Answer from the drawing. Dimensions are ordinates in mm from the lowest x, y and z of the part. A direction names the side the tool comes from. Round coordinates to 2 decimals unless told otherwise and drop trailing zeros. Loops run counter-clockwise (first coordinate to the right, second up) from the corner with the lowest first, then second, coordinate; pieces in that order, holes last. Notation, with made-up numbers: (-40, -29.75) - (-18, -29.75) arc R29 cw to (-18, -6.75) - close; hole circle Ø9 at (-27, 18.25). An arc over 180 degrees is marked (long way). Write item = value, one per line. Start each with the question number.
1) For a pull along X with two mould halves and no side action, classify the marked faces 1, 2, 3 and 4 as released by +X, released by -X, zero draft, split by the parting line, or undercut.
2) Section D-D, the plane y = 23.5 is taken. Determine the outline of the cut face in (x, z).
3) A tool of negligible diameter and unlimited length cuts with its end or side. For the marked faces 5 and 6, from which of +Z, -Z, +X, -X, +Y, -Y can it reach the whole face along a straight path? Write none if from no direction.
4) Given pin 1 Ø1.5 at (x, z) = (55, 13.5) entering from -Y; pin 2 Ø10 at (y, z) = (11.5, 63) entering from +X; pin 3 Ø2 at (y, z) = (15.5, 43.5) entering from +X (1 decimal), each flat-ended and moving along its own axis, determine where each tip first touches the part or whether it passes through.
5) Straight lines are drawn through the part: line 1 along Z through (x, y) = (50.8, 34.5); line 2 along Z through (x, y) = (50.8, 15.5); line 3 along Y through (x, z) = (118, 14.5). For each, find the intervals that lie inside material, in ascending order.
6) Section B-B, the plane x = 27 is taken. Determine the outline of the cut face in (y, z).
7) Section C-C, the plane y = 41.5 is taken. Determine the outline of the cut face in (x, z).
8) Section A-A, the plane z = 50.8 is taken. Determine the outline of the cut face in (x, y), and give its area (3 significant figures).
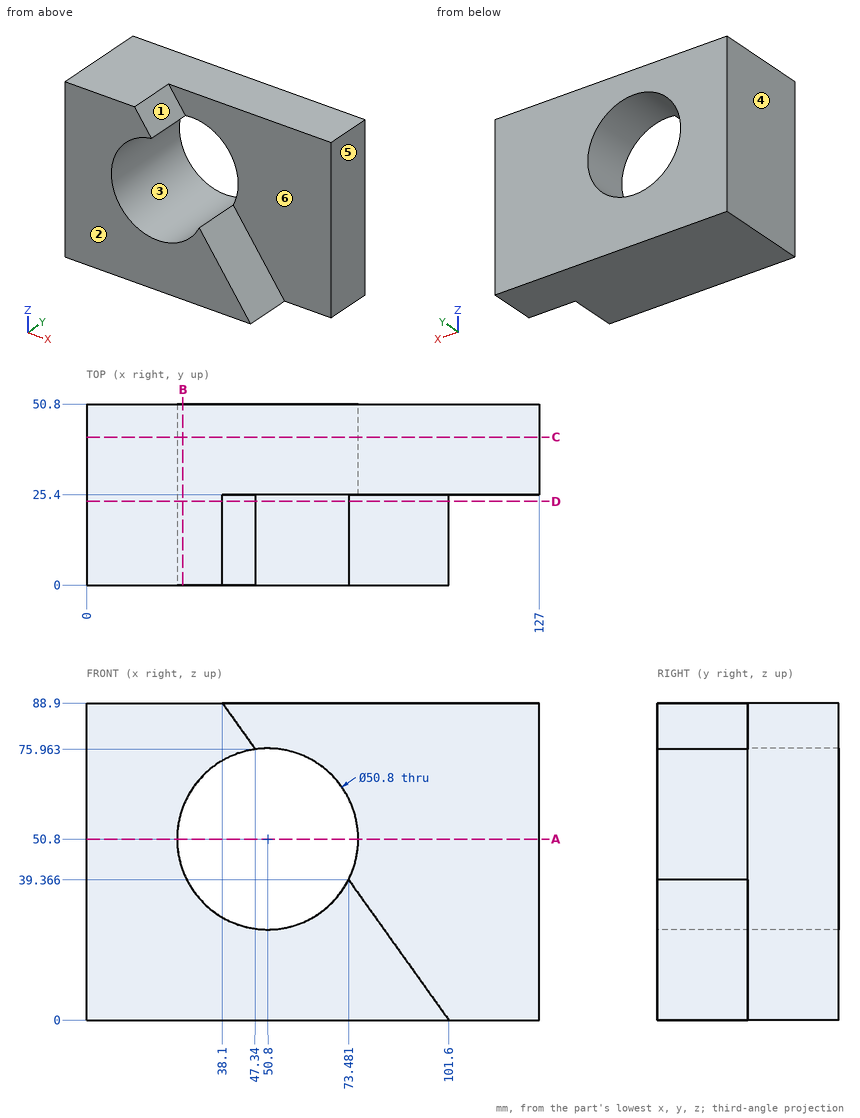
Geometry check:
q1.face_1 = released by +X
q1.face_2 = zero draft
q1.face_3 = undercut
q1.face_4 = released by -X
q2.outline = (0, 0) - (101.6, 0) - (73.48, 39.37) arc R25.4 cw (long way) to (47.34, 75.96) - (38.1, 88.9) - (0, 88.9) - close
q3.face_5 = +Z, -Z, +X, +Y, -Y
q3.face_6 = +Z, +X, -Y
q4.pin_1 = 0
q4.pin_2 = 32.11
q4.pin_3 = 26.8
q5.line_1 = 0 to 25.4, 76.2 to 88.9
q5.line_2 = 0 to 25.4
q5.line_3 = 25.4 to 50.8
q6.outline = (0, 0) - (50.8, 0) - (50.8, 41.93) - (0, 41.93) - close; (0, 59.67) - (50.8, 59.67) - (50.8, 88.9) - (0, 88.9) - close
q7.outline = (0, 0) - (127, 0) - (127, 88.9) - (0, 88.9) - close; hole circle Ø50.8 at (50.8, 50.8)
q8.outline = (0, 0) - (25.4, 0) - (25.4, 50.8) - (0, 50.8) - close; (76.2, 25.4) - (127, 25.4) - (127, 50.8) - (76.2, 50.8) - close
q8.area = 2,580 mm2
